from build123d import *

# Parameters (mm, degrees)
SALIENTE_EXTRUIR1_DEPTH = 20
CORTAR_EXTRUIR1_DEPTH   = 8
CROQUIS3_W              = 20
CROQUIS3_H              = 20
SALIENTE_EXTRUIR2_DEPTH = 20


with BuildPart() as part:
    # Croquis1 → Saliente-Extruir1 (new body)
    with BuildSketch(Plane.XY):
        with BuildLine():
            Line((0, 90), (0, 10))
            Line((0, 10), (17.5, 10))
            ThreePointArc((17.5, 10), (20, 12.5), (22.5, 10))
            Line((22.5, 10), (40, 10))
            Line((40, 10), (40, 90))
            ThreePointArc((40, 90), (37.071067812, 97.071067812), (30, 100))
            Line((30, 100), (10, 100))
            ThreePointArc((10, 100), (2.928932188, 97.071067812), (0, 90))
        make_face()
        with BuildLine():
            Line((17.5, 10), (0, 10))
            ThreePointArc((0, 10), (2.928932188, 2.928932188), (10, 0))
            Line((10, 0), (30, 0))
            ThreePointArc((30, 0), (37.071067812, 2.928932188), (40, 10))
            Line((40, 10), (22.5, 10))
            ThreePointArc((22.5, 10), (22.371708245, 9.209430585), (22, 8.5))
            ThreePointArc((22, 8.5), (20, 7.5), (18, 8.5))
            ThreePointArc((18, 8.5), (17.628291755, 9.209430585), (17.5, 10))
        make_face()
        with BuildLine():
            ThreePointArc((22.5, 10), (20, 12.5), (17.5, 10))
            ThreePointArc((17.5, 10), (17.628291755, 9.209430585), (18, 8.5))
            Line((18, 8.5), (22, 8.5))
            ThreePointArc((22, 8.5), (22.371708245, 9.209430585), (22.5, 10))
        make_face()
        with BuildLine():
            Line((22, 8.5), (18, 8.5))
            ThreePointArc((18, 8.5), (20, 7.5), (22, 8.5))
        make_face()
    extrude(amount=SALIENTE_EXTRUIR1_DEPTH)

    # Croquis2 → Cortar-Extruir1 (cut)
    with BuildSketch(Plane(origin=(0, 0, 0), x_dir=(-1, 0, 0), z_dir=(0, 0, -1))):
        with BuildLine():
            Line((-22, 8.5), (-20, 8.5))
            Line((-20, 8.5), (-18, 8.5))
            ThreePointArc((-18, 8.5), (-17.628291755, 9.209430585), (-17.5, 10))
            ThreePointArc((-17.5, 10), (-20.790569415, 12.371708245), (-22, 8.5))
        make_face()
    extrude(amount=-CORTAR_EXTRUIR1_DEPTH, mode=Mode.SUBTRACT)

    # Croquis3 → Saliente-Extruir2 (add)
    with BuildSketch(Plane(origin=(0, 100, 0), x_dir=(1, 0, 0), z_dir=(0, 1, 0))):
        with Locations((20, -30)):
            Rectangle(CROQUIS3_W, CROQUIS3_H)
    extrude(amount=-SALIENTE_EXTRUIR2_DEPTH)


solid = part.part
Read the model definition and answer for the solid it produces. Units are mm, in the model's axes. A direction names the side the tool comes from. Round coordinates to 2 decimals unless told otherwise and drop trailing zeros. Loops run counter-clockwise (first coordinate to the right, second up) from the corner with the lowest first, then second, coordinate; pieces in that order, holes last.
Q1. Section B-B on z = 9.5 is taken. Write down the section's boundary in (x, y).
Q2. Which of the six approach directions +Z, -Z, +X, -X, +Y, -Y give full straight-line access (tool end or side, diameter ignored) to faces 1 (the face through (2.85, 3.01, 9.86)), 2 (the face through (20, 8.5, 4)), 3 (the face through (10, 90, 30))?
Q3. Each of these flat-tipped pins is pushed along its axis until it touches: pin 1 (10 mm diameter, centred on x = 15.5, z = 28.5, fed in from -Y); pin 2 (10 mm diameter, centred on y = 90, z = 34.5, fed in from -X); pin 3 (6 mm diameter, centred on y = 94, z = 32, fed in from +X). Where does it stop, or does it pass through?
Q4. Determine the mould class of faces 4 (the face through (20, 11, 8)), 5 (the face through (3.01, 97.15, 9.86)), 6 (the face through (20, 80, 30)), 7 (the face through (30, 90, 30)) for opening direction X: released by +X, released by -X, zero draft, split by the parting line, or undercut.
Q5. Consider probe 1 along X at (y, z) = (10, 6); probe 2 along Y at (x, z) = (20, 5); probe 3 along Z at (x, y) = (4, 22). Determine where each line is inside the solid, lowest interval first.
Q6. Section C-C on x = 20 is taken. Write down the section's boundary in (y, z), and give its area (3 significant figures).
Q7. Section D-D on x = 25.5 is taken. Write down the section's boundary in (y, z).
Q8. Section A-A on y = 81.5 is taken. Write down the section's boundary in (x, z), and give its area (3 significant figures).
Output:
1. outline: (0, 10) arc R10 ccw to (10, 0) - (30, 0) arc R10 ccw to (40, 10) - (40, 90) arc R10 ccw to (30, 100) - (10, 100) arc R10 ccw to (0, 90) - close
2. face 1: +Z, -Z, -X, -Y
2. face 2: -Z
2. face 3: +Z, -X, +Y, -Y
3. pin 1: stops at y = 80
3. pin 2: stops at x = 10
3. pin 3: stops at x = 30
4. face 4: undercut
4. face 5: released by -X
4. face 6: zero draft
4. face 7: released by +X
5. probe 1: x = 0 to 17.5, 22.5 to 40
5. probe 2: y = 0 to 8.5, 12.5 to 100
5. probe 3: z = 0 to 20
6. outline: (0, 0) - (8.5, 0) - (8.5, 8) - (12.5, 8) - (12.5, 0) - (100, 0) - (100, 40) - (80, 40) - (80, 20) - (0, 20) - close
6. area: 2,370 mm2
7. outline: (0, 0) - (100, 0) - (100, 40) - (80, 40) - (80, 20) - (0, 20) - close
8. outline: (0, 0) - (40, 0) - (40, 20) - (30, 20) - (30, 40) - (10, 40) - (10, 20) - (0, 20) - close
8. area: 1,200 mm2
